from build123d import *

# Parameters (mm, degrees)
SKETCH1_W                      = 6.5
SKETCH1_H                      = 9
BOSS_EXTRUDE1_DEPTH            = 150
BOSS_EXTRUDE2_DEPTH            = 14.45
M3X0_5_TAPPED_HOLE1_AT_2_COUNT = 2
M3X0_5_TAPPED_HOLE1_AT_2_PITCH = 18.027756377
M3X0_5_TAPPED_HOLE1_AT_3_COUNT = 2
M3X0_5_TAPPED_HOLE1_AT_3_PITCH = 15
M3X0_5_TAPPED_HOLE1_AT_4_COUNT = 2
M3X0_5_TAPPED_HOLE1_AT_4_PITCH = 10
LPATTERN1_COUNT                = 15
LPATTERN1_PITCH                = 20


with BuildPart() as part:
    # Sketch1 → Boss-Extrude1 (new body, symmetric)
    with BuildSketch(Plane.XY):
        Rectangle(SKETCH1_W, SKETCH1_H)
    extrude(amount=BOSS_EXTRUDE1_DEPTH, both=True)

    # Sketch6 → CBORE for M3 SHCS1 (revolve, cut)
    with BuildSketch(Plane(origin=(-3.25, 0, -140), x_dir=(0, 0, 1), z_dir=(0, 1, 0))):
        Polygon((0, 0), (0, 6.5), (1.8, 6.5), (1.8, 3), (3.25, 3), (3.25, 0), align=None)
    cbore_for_m3_shcs1 = revolve(axis=Axis((-9.6, 0, -140), (1, 0, 0)), mode=Mode.SUBTRACT)

    # LPattern1: CBORE for M3 SHCS1 ×15
    with Locations(*[(0, 0, i * LPATTERN1_PITCH) for i in range(1, LPATTERN1_COUNT)]):
        add(cbore_for_m3_shcs1, mode=Mode.SUBTRACT)


with BuildPart() as body_2:
    # Sketch2 → Boss-Extrude2 (new body, symmetric)
    with BuildSketch(Plane.XY):
        Polygon((0.75, 4.75), (0.75, 10), (-7.25, 10), (-7.25, -10), (0.75, -10), (0.75, -4.75), (-3.45, -4.75), (-3.45, 4.75), align=None)
    extrude(amount=BOSS_EXTRUDE2_DEPTH, both=True)

    # Sketch4 → M3x0.5 Tapped Hole1 (revolve, cut)
    with BuildSketch(Plane(origin=(-7.25, 7.5, -5), x_dir=(0, 0, 1), z_dir=(0, 1, 0))):
        Polygon((0, 0), (0, 3.751075774), (1.25, 3), (1.25, 0), align=None)
    m3x0_5_tapped_hole1 = revolve(axis=Axis((-13.6, 7.5, -5), (1, 0, 0)), mode=Mode.SUBTRACT)

    # M3x0.5 Tapped Hole1 at 2: M3x0.5 Tapped Hole1 ×2
    with Locations(*[Vector(0, -0.832050294, 0.554700196) * (i * M3X0_5_TAPPED_HOLE1_AT_2_PITCH) for i in range(1, M3X0_5_TAPPED_HOLE1_AT_2_COUNT)]):
        add(m3x0_5_tapped_hole1, mode=Mode.SUBTRACT)

    # M3x0.5 Tapped Hole1 at 3: M3x0.5 Tapped Hole1 ×2
    with Locations(*[(0, -i * M3X0_5_TAPPED_HOLE1_AT_3_PITCH, 0) for i in range(1, M3X0_5_TAPPED_HOLE1_AT_3_COUNT)]):
        add(m3x0_5_tapped_hole1, mode=Mode.SUBTRACT)

    # M3x0.5 Tapped Hole1 at 4: M3x0.5 Tapped Hole1 ×2
    with Locations(*[(0, 0, i * M3X0_5_TAPPED_HOLE1_AT_4_PITCH) for i in range(1, M3X0_5_TAPPED_HOLE1_AT_4_COUNT)]):
        add(m3x0_5_tapped_hole1, mode=Mode.SUBTRACT)


with BuildPart() as body_2_1:
    # Body-Move/Copy1: moved
    add(body_2.part.moved(Location((0, 0, 5))))


solid = body_2_1.part
For this review, take the finished solid that the model builds, in its own axes (mm). A direction names the side the tool comes from. Give positions to 0.01 mm unless a question says otherwise; leave off trailing zeros. Order: outer loops, then holes, each group sorted by start corner. A loop starts at its lowest first (then second) coordinate and runs counter-clockwise, first axis right, second up. Notation, with made-up numbers: (25, -19.5) -> (70, -19.5) arc R30 cw to (70, 5.5) -> close; hole circle Ø3 at (47, -34). An arc over 180 degrees is marked (long way). Write item = value, one per line.
1) We need section B-B, the plane z = 7.75. Give the boundary of the cut face in (x, y).
Findings:
outline = (-7.25, -10) -> (0.75, -10) -> (0.75, -4.75) -> (-3.45, -4.75) -> (-3.45, 4.75) -> (0.75, 4.75) -> (0.75, 10) -> (-7.25, 10) -> close
2) We need section C-C, the plane y = -2. Give the boundary of the cut face in (x, z).
Findings:
outline = (-7.25, -9.45) -> (-3.45, -9.45) -> (-3.45, 19.45) -> (-7.25, 19.45) -> close
3) Insertion check: pin 1 (2 mm diameter, centred on y = 7.5, z = 10, fed in from -X). The pin has a flat end and moves straight along its axis. Give the tip position at first contact, or say it passes through.
Findings:
pin_1 = -4.1
4) Draft analysis for pull direction Z (two halves, no side actions). For faces 4 (the face through (-5.77, 7.45, 8.75)), 5 (the face through (-1, -4.75, 5)), 6 (the face through (-4, 0, -9.45)), 7 (the face through (-5.77, 8.72, -0.27)), state which applies: pulls with the +Z half, pulls with the -Z half, needs draft (parallel to the pull), parting line crosses it, or undercut.
Findings:
face_4 = undercut
face_5 = needs draft
face_6 = pulls with the -Z half
face_7 = undercut
5) To check wall thickness, follow L1, parallel to Y at x = -5.1, z = 10; L2, parallel to Z at x = -6.15, y = 7.5; L3, parallel to Y at x = -3, z = 2.5. State the ranges of each line that lie inside material, in increasing order. Write a range as from..to.
Findings:
L1 = -10..-8.75, -6.25..6.25, 8.75..10
L2 = -9.45..-1.25, 1.25..8.75, 11.25..19.45
L3 = -10..-4.75, 4.75..10
6) For faces 1 (the face through (-5.77, -6.28, -0.27)), 2 (the face through (-1, 4.75, 5)), 3 (the face through (-3, 10, 5)), list the 3-axis set-ups (+Z, -Z, +X, -X, +Y, -Y) from which the entire face can be reached by the end or side of a thin tool; tool diameter is ignored.
Findings:
face_1 = -X
face_2 = +Z, -Z, +X
face_3 = +Z, -Z, +X, -X, +Y
7) We need section A-A, the plane x = 0.25. Give the boundary of the cut face in (y, z), and give its area (3 significant figures).
Findings:
outline = (-10, -9.45) -> (-4.75, -9.45) -> (-4.75, 19.45) -> (-10, 19.45) -> close; (4.75, -9.45) -> (10, -9.45) -> (10, 19.45) -> (4.75, 19.45) -> close
area = 303 mm^2
